Design review of the part built by this model. Coordinates are the model's own, in mm. Face numbers are marked on the shaded views. Coordinates: 2 decimals unless noted, no trailing zeros. Order: outer loops, then holes, each group sorted by start corner. A loop starts at its lowest first (then second) coordinate and runs counter-clockwise, first axis right, second up. Notation, with made-up numbers: (80.25, -31) -> (84.25, -31) arc R12 ccw to (84.25, -14) -> close; hole circle Ø10 at (-25, 3.25). An arc over 180 degrees is marked (long way). Write item = value, one per line.
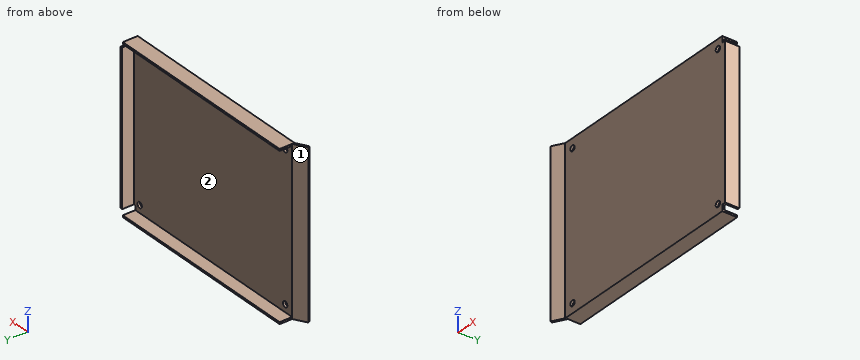
```python
from build123d import *

# Parameters (mm, degrees)
BOSS_EXTRUDE1_DEPTH = 130
SKETCH3_W           = 3
SKETCH3_H           = 5
CUT_EXTRUDE1_DEPTH  = 12.5
SKETCH4_W           = 161.719208284
SKETCH4_H           = 1.5
BOSS_EXTRUDE2_DEPTH = 10
SKETCH5_R           = 2.25
CUT_EXTRUDE2_DEPTH  = 7.945980836
FILLET1_R           = 0.5


with BuildPart() as part:
    # Sketch1 → Boss-Extrude1 (new body)
    with BuildSketch(Plane.XY):
        Polygon((-4.857650715, 2.326869046), (-14.638442431, -3.320073684), (-13.888442431, -4.61911179), (-5.138442431, 0.432703066), (159.861557569, 0.432703066), (159.861557569, 11.932703066), (158.361557569, 11.932703066), (158.361557569, 2.326869046), align=None)
    extrude(amount=BOSS_EXTRUDE1_DEPTH)

    # Sketch3 → Cut-Extrude1 (cut, through all)
    with BuildSketch(Plane.XZ.offset(-0.432703066)):
        with Locations((158.361557569, 127.5)):
            Rectangle(SKETCH3_W, SKETCH3_H)
        with Locations((158.361557569, 2.5)):
            Rectangle(SKETCH3_W, SKETCH3_H)
    extrude(amount=-CUT_EXTRUDE1_DEPTH, mode=Mode.SUBTRACT)

    # Sketch4 → Boss-Extrude2 (add)
    with BuildSketch(Plane(origin=(0, 2.326869046, 0), x_dir=(1, 0, 0), z_dir=(0, 1, 0))):
        with Locations((76.001953427, -129.25)):
            Rectangle(SKETCH4_W, SKETCH4_H)
        with Locations((76.001953427, -0.75)):
            Rectangle(SKETCH4_W, SKETCH4_H)
    extrude(amount=BOSS_EXTRUDE2_DEPTH)

    # Sketch5 → Cut-Extrude2 (cut, through all)
    with BuildSketch(Plane(origin=(0, 2.326869046, 0), x_dir=(1, 0, 0), z_dir=(0, 1, 0))):
        with Locations((2.361557569, -122.5)):
            Circle(SKETCH5_R)
        with Locations((2.361557569, -7.5)):
            Circle(SKETCH5_R)
        with Locations((152.361557569, -7.5)):
            Circle(SKETCH5_R)
        with Locations((152.361557569, -122.5)):
            Circle(SKETCH5_R)
    extrude(amount=-CUT_EXTRUDE2_DEPTH, mode=Mode.SUBTRACT)

    # Fillet1
    fillet1_edges = [part.edges().sort_by_distance(p)[0] for p in [
        (-14.263442431, -3.969592737, 130),
        (159.111557569, 11.932703066, 125),
        (159.111557569, 11.932703066, 5),
        (-4.857650715, 2.326869046, 65),
        (156.861557569, 12.326869046, 129.25),
        (-4.857650715, 12.326869046, 129.25),
        (-4.857650715, 12.326869046, 0.75),
        (156.861557569, 12.326869046, 0.75),
        (-14.263442431, -3.969592737, 0),
    ]]
    fillet(fillet1_edges, radius=FILLET1_R)


solid = part.part
```
(1) Insertion check: pin 1 (1.5 mm diameter, centred on y = 4.5, z = 128, fed in from +X); pin 2 (3.5 mm diameter, centred on x = 159, y = 5.5, fed in from +Z); pin 3 (5 mm diameter, centred on x = 152.36, z = 7.5, fed in from +Y). Each pin has a flat end and moves straight along its axis. Give the tip position at first contact, or say it passes through.
Report:
pin_1 = 156.86
pin_2 = 125
pin_3 = 2.33
(2) We need section C-C (z = 80). Write out the cut boundary in (x, y), and give its area (3 significant figures).
Report:
outline = (-14.64, -3.32) -> (-13.89, -4.62) -> (-5.14, 0.43) -> (159.86, 0.43) -> (159.86, 11.93) -> (158.36, 11.93) -> (158.36, 2.33) -> (-4.72, 2.33) arc R0.5 ccw to (-4.97, 2.26) -> close
area = 343 mm²
(3) The part is to be moulded in two halves that separate along Z. For the marked faces 1 and 2, say which applies: released by +Z, released by -Z, zero draft, split by the parting line, or undercut.
Report:
face_1 = zero draft
face_2 = undercut
(4) We need section A-A (z = 7.5). Write out the cut boundary in (x, y).
Report:
outline = (-14.64, -3.32) -> (-13.89, -4.62) -> (-5.14, 0.43) -> (0.11, 0.43) -> (0.11, 2.33) -> (-4.72, 2.33) arc R0.5 ccw to (-4.97, 2.26) -> close; (4.61, 0.43) -> (150.11, 0.43) -> (150.11, 2.33) -> (4.61, 2.33) -> close; (154.61, 0.43) -> (159.86, 0.43) -> (159.86, 11.93) -> (158.36, 11.93) -> (158.36, 2.33) -> (154.61, 2.33) -> close
(5) We need section B-B (x = 49.5). Write out the cut boundary in (y, z).
Report:
outline = (0.43, 0) -> (12.33, 0) -> (12.33, 1.5) -> (2.33, 1.5) -> (2.33, 128.5) -> (12.33, 128.5) -> (12.33, 130) -> (0.43, 130) -> close
(6) For L1, parallel to Z at x = 118, y = 10.5; L2, parallel to X at y = 1.15, z = 7.5; L3, parallel to X at y = 1.7, z = 7.5, list the stretches that pass through material, from the lowest coordinate up.
Report:
L1 = 0 to 1.5, 128.5 to 130
L2 = -6.9 to 0.11, 4.61 to 150.11, 154.61 to 159.86
L3 = -5.94 to 0.11, 4.61 to 150.11, 154.61 to 159.86
